Autodesk Inventor part; units mm, degrees
ref_plane "FP_XY" through (0, 0, 0) normal (0, -1, 0) x (1, 0, 0)
ref_plane "FP_YZ" through (0, 0, 0) normal (1, 0, 0) x (0, 0, 1)
ref_plane "FP_ZX" through (0, 0, 0) normal (0, 0, 1) x (0, -1, 0)
sketch "Sketch_4" plane through (0, 0, 0) normal (0, 1, 0) x (1, 0, 0)
  arc A0 (-223.5, -42.5) -> (-191.5, -74.5) centre (-191.5, -42.5) ccw
  line L0 (-191.5, -74.5) -> (191.5, -74.5)
  arc A1 (191.5, -74.5) -> (223.5, -42.5) centre (191.5, -42.5) ccw
  line L1 (223.5, -42.5) -> (223.5, 42.5)
  arc A2 (223.5, 42.5) -> (191.5, 74.5) centre (191.5, 42.5) ccw
  line L2 (191.5, 74.5) -> (-191.5, 74.5)
  arc A3 (-191.5, 74.5) -> (-223.5, 42.5) centre (-191.5, 42.5) ccw
  line L3 (-223.5, 42.5) -> (-223.5, -42.5)
  circle A4 centre (215.5, 0) radius 3.6
  circle A5 centre (174, -66.5) radius 3.6
  circle A6 centre (174, 66.5) radius 3.6
  circle A7 centre (60, -66.5) radius 3.6
  circle A8 centre (60, 66.5) radius 3.6
  circle A9 centre (-60, -66.5) radius 3.6
  circle A10 centre (-60, 66.5) radius 3.6
  circle A11 centre (-174, -66.5) radius 3.6
  circle A12 centre (-174, 66.5) radius 3.6
  circle A13 centre (-215.5, 0) radius 3.6
extrude "Extrusion1" add sketch "Sketch_4" along normal blind 1.5
ref_plane "FP_XY" through (0, 0, 0) normal (0, -1, 0) x (1, 0, 0)
ref_plane "FP_YZ" through (0, 0, 0) normal (1, 0, 0) x (0, 0, 1)
ref_plane "FP_ZX" through (0, 0, 0) normal (0, 0, 1) x (0, -1, 0)
ref_plane "to_Bolt_1_XY" through (-215.5, 0, 0) normal (0, 1, 0) x (1, 0, 0)
ref_plane "to_Bolt_1_YZ" through (-215.5, 0, 0) normal (1, 0, 0) x (0, 0, -1)
ref_plane "to_Bolt_1_ZX" through (-215.5, 0, 0) normal (0, 0, -1) x (0, 1, 0)
ref_plane "to_Bolt_1_1_XY" through (-174, 0, -66.5) normal (0, 1, 0) x (1, 0, 0)
ref_plane "to_Bolt_1_1_YZ" through (-174, 0, -66.5) normal (1, 0, 0) x (0, 0, -1)
ref_plane "to_Bolt_1_1_ZX" through (-174, 0, -66.5) normal (0, 0, -1) x (0, 1, 0)
ref_plane "to_Bolt_1_2_XY" through (-60, 0, -66.5) normal (0, 1, 0) x (1, 0, 0)
ref_plane "to_Bolt_1_2_YZ" through (-60, 0, -66.5) normal (1, 0, 0) x (0, 0, -1)
ref_plane "to_Bolt_1_2_ZX" through (-60, 0, -66.5) normal (0, 0, -1) x (0, 1, 0)
ref_plane "to_Bolt_1_3_XY" through (60, 0, -66.5) normal (0, 1, 0) x (1, 0, 0)
ref_plane "to_Bolt_1_3_YZ" through (60, 0, -66.5) normal (1, 0, 0) x (0, 0, -1)
ref_plane "to_Bolt_1_3_ZX" through (60, 0, -66.5) normal (0, 0, -1) x (0, 1, 0)
ref_plane "to_Bolt_1_4_XY" through (174, 0, -66.5) normal (0, 1, 0) x (1, 0, 0)
ref_plane "to_Bolt_1_4_YZ" through (174, 0, -66.5) normal (1, 0, 0) x (0, 0, -1)
ref_plane "to_Bolt_1_4_ZX" through (174, 0, -66.5) normal (0, 0, -1) x (0, 1, 0)
ref_plane "to_Bolt_1_5_XY" through (-174, 0, 66.5) normal (0, 1, 0) x (1, 0, 0)
ref_plane "to_Bolt_1_5_YZ" through (-174, 0, 66.5) normal (1, 0, 0) x (0, 0, -1)
ref_plane "to_Bolt_1_5_ZX" through (-174, 0, 66.5) normal (0, 0, -1) x (0, 1, 0)
ref_plane "to_Bolt_1_6_XY" through (-60, 0, 66.5) normal (0, 1, 0) x (1, 0, 0)
ref_plane "to_Bolt_1_6_YZ" through (-60, 0, 66.5) normal (1, 0, 0) x (0, 0, -1)
ref_plane "to_Bolt_1_6_ZX" through (-60, 0, 66.5) normal (0, 0, -1) x (0, 1, 0)
ref_plane "to_Bolt_1_7_XY" through (60, 0, 66.5) normal (0, 1, 0) x (1, 0, 0)
ref_plane "to_Bolt_1_7_YZ" through (60, 0, 66.5) normal (1, 0, 0) x (0, 0, -1)
ref_plane "to_Bolt_1_7_ZX" through (60, 0, 66.5) normal (0, 0, -1) x (0, 1, 0)
ref_plane "to_Bolt_1_8_XY" through (174, 0, 66.5) normal (0, 1, 0) x (1, 0, 0)
ref_plane "to_Bolt_1_8_YZ" through (174, 0, 66.5) normal (1, 0, 0) x (0, 0, -1)
ref_plane "to_Bolt_1_8_ZX" through (174, 0, 66.5) normal (0, 0, -1) x (0, 1, 0)
ref_plane "to_Bolt_2_XY" through (215.5, 0, 0) normal (0, 1, 0) x (1, 0, 0)
ref_plane "to_Bolt_2_YZ" through (215.5, 0, 0) normal (1, 0, 0) x (0, 0, -1)
ref_plane "to_Bolt_2_ZX" through (215.5, 0, 0) normal (0, 0, -1) x (0, 1, 0)
properties part number "1XX4_04_00_4(1)_P5"
Here's how the part is built. I have some questions about the finished solid (model axes, mm). Coordinates: 2 decimals unless noted, no trailing zeros. Use one line per item in the form item = value. Start each with the question number.
(1) Please list where these lines run through material, in increasing order: line 1 along Z through (x, y) = (-174, 1.1); line 2 along X through (y, z) = (0.45, 0); line 3 along X through (y, z) = (1.3, -66.5).
(2) If we section it at A-A (y = 1.25): Give the number of separate pieces and of enclosed holes in the cut face, then the cut area to 3 significant figures.
(3) We'd pull the mould along X, two halves only. Please class faces 1 (the face through (171.347, 0.74, -64.067)), 2 (the face through (-3, 0, -1)), 3 (the face through (213.88, 0.74, -65.37)), 4 (the face through (211.903, 0.74, 0.158)): pulls with the +X half, pulls with the -X half, needs draft (parallel to the pull), parting line crosses it, or undercut.
Verdict:
q1.line_1 = -74.5 to -70.1, -62.9 to 62.9, 70.1 to 74.5
q1.line_2 = -223.5 to -219.1, -211.9 to 211.9, 219.1 to 223.5
q1.line_3 = -212.67 to -177.6, -170.4 to -63.6, -56.4 to 56.4, 63.6 to 170.4, 177.6 to 212.67
q2.separate_pieces = 1
q2.enclosed_holes = 10
q2.area = 65,300 mm²
q3.face_1 = undercut
q3.face_2 = needs draft
q3.face_3 = pulls with the +X half
q3.face_4 = undercut
